The listing builds one solid part. Answer for the finished solid, in the listing's coordinates (mm). A direction names the side the tool comes from. Coordinates: 2 decimals unless noted, no trailing zeros. Answer as a JSON object with one key per item and string values. Group by question number.
1. Straight lines are drawn through the part: L1, parallel to Z at x = 26, y = -15.5; L2, parallel to X at y = -50, z = -3. For each, find the intervals that lie inside material, in ascending order.
2. A cutting plane is placed at A-A on z = -32. State how many separate pieces and enclosed holes the cut face has, and give its area (3 significant figures).
3. For faces 1 (the face through (0, -39, 0)), 2 (the face through (-26.997, -39.44, -20.21)), determine the directions among +Z, -Z, +X, -X, +Y, -Y from which every point of the face is accessible in a straight line to the end or side of a thin tool.
4. Given pin 1 (2 mm diameter, centred on y = -53.5, z = -18.5, fed in from +X); pin 2 (0.5 mm diameter, centred on x = -5, y = -55, fed in from -Z); pin 3 (6 mm diameter, centred on y = -14, z = -7, fed in from +X), each flat-ended and moving along its own axis, determine where each tip first touches the part or whether it passes through.
from build123d import *

# Parameters (mm, degrees)
BOSS_EXTRUDE1_DEPTH = 80


with BuildPart() as part:
    # Sketch1 → Boss-Extrude1 (new body)
    with BuildSketch(Plane(origin=(0, 0, 0), x_dir=(1, 0, 0), z_dir=(0, 1, 0))):
        Polygon((0, 5), (0, 0), (30.606505653, 0), (30.344466757, 5), (28.772233378, 35), (27.772233378, 35), (26.2, 5), (25.704466757, 5), (25.7, 5), (25.204466757, 5), (23.632233378, 35), (22.632233378, 35), (21.06, 5), (20.564466757, 5), (20.56, 5), (20.064466757, 5), (18.492233378, 35), (17.492233378, 35), (15.92, 5), (15.424466757, 5), (15.42, 5), (14.924466757, 5), (13.352233378, 35), (12.352233378, 35), (10.78, 5), (10.284466757, 5), (10.28, 5), (9.784466757, 5), (8.212233378, 35), (7.212233378, 35), (5.64, 5), (5.144466757, 5), (5.14, 5), (4.644466757, 5), (3.072233378, 35), (2.072233378, 35), (0.5, 5), align=None)
    boss_extrude1 = extrude(amount=-BOSS_EXTRUDE1_DEPTH)

    # Mirror1: Boss-Extrude1 across plane
    add(boss_extrude1.mirror(Plane(origin=(0, -80, 0), x_dir=(0, 0, 1), z_dir=(1, 0, 0))))


solid = part.part
From the geometry:
{
 "1": {"L1": "z = -5 to 0", "L2": "x = -30.45 to 30.45"},
 "2": {"separate pieces": "12", "enclosed holes": "0", "area": "1,260 mm²"},
 "3": {"face 1": "+Z, +X, -X, +Y, -Y", "face 2": "-Z, +Y, -Y"},
 "4": {"pin 1": "stops at x = 29.69", "pin 2": "stops at z = -5", "pin 3": "stops at x = 30.4"}
}
